Build history of the part. All positions in model axes, mm. Give positions to 0.01 mm unless a question says otherwise; leave off trailing zeros. Write each loop counter-clockwise with the first axis right and the second up, starting at its lowest first coordinate (ties: lowest second). Pieces come first, ordered by that corner, then holes.
from build123d import *

# Parameters (mm, degrees)
BOSS_EXTRUDE1_DEPTH = 1
BOSS_EXTRUDE2_DEPTH = 1.5
SKETCH3_W           = 70
SKETCH3_H           = 40
CUT_EXTRUDE1_DEPTH  = 10
SKETCH4_R           = 2.25
SKETCH4_R_2         = 3.25
CUT_EXTRUDE3_DEPTH  = 10


with BuildPart() as part:
    # Sketch1 → Boss-Extrude1 (new body)
    with BuildSketch(Plane.XY):
        Polygon((-85, 42), (85, 42), (86.5, 0), (85, -42), (-85, -42), (-86.5, 0), align=None)
    extrude(amount=BOSS_EXTRUDE1_DEPTH)

    # Sketch2 → Boss-Extrude2 (add)
    with BuildSketch(Plane.XY.offset(1)):
        Polygon((-83, 40.25), (83, 40.25), (84.5, 0), (83, -40.25), (-83, -40.25), (-84.5, 0), align=None)
    extrude(amount=BOSS_EXTRUDE2_DEPTH)

    # Sketch3 → Cut-Extrude1 (cut)
    with BuildSketch(Plane(origin=(0, 0, 0), x_dir=(-1, 0, 0), z_dir=(0, 0, -1))):
        with Locations((-27.5, 12)):
            Rectangle(SKETCH3_W, SKETCH3_H)
    extrude(amount=-CUT_EXTRUDE1_DEPTH, mode=Mode.SUBTRACT)

    # Sketch4 → Cut-Extrude3 (cut)
    with BuildSketch(Plane(origin=(0, 0, 0), x_dir=(-1, 0, 0), z_dir=(0, 0, -1))):
        with Locations((-65.954695658, -30.705934388)):
            Circle(SKETCH4_R)
        with Locations((-45.954695658, -30.705934388)):
            Circle(SKETCH4_R)
        with Locations((-9.054695658, -30.705934388)):
            Circle(SKETCH4_R)
        with Locations((10.945304342, -30.705934388)):
            Circle(SKETCH4_R)
        with Locations((47.845022936, -30.705934388)):
            Circle(SKETCH4_R)
        with Locations((67.845022936, -30.705934388)):
            Circle(SKETCH4_R)
        with Locations((67.845022936, -3.141963924)):
            Circle(SKETCH4_R)
        with Locations((47.845022936, -3.141963924)):
            Circle(SKETCH4_R)
        with Locations((57.845022936, 25.044065612)):
            Circle(SKETCH4_R_2)
    extrude(amount=-CUT_EXTRUDE3_DEPTH, mode=Mode.SUBTRACT)


solid = part.part
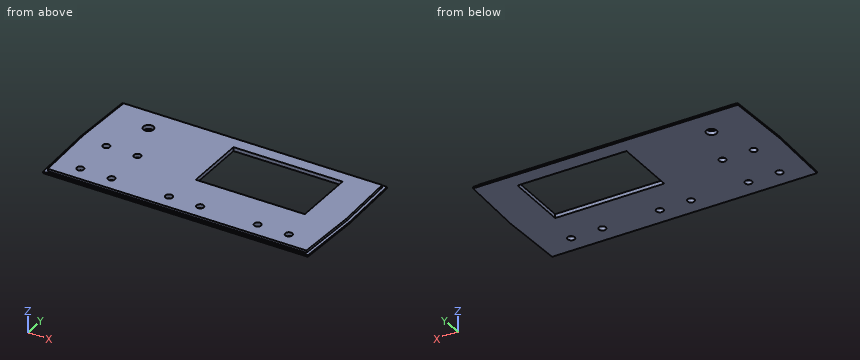
1. Drop flat-ended pins along their axis: pin 1 (0.8 mm diameter, centred on x = -26, z = 2, fed in from -Y); pin 2 (1 mm diameter, centred on x = 11.5, z = 2, fed in from +Y); pin 3 (0.8 mm diameter, centred on y = 6.5, z = 1.5, fed in from -X). Give the stop position or say it passes through.
2. Drill centre lines: line 1 along Y through (x, z) = (60.5, 1.65); line 2 along Y through (x, z) = (26.5, 0.6); line 3 along Y through (x, z) = (-68, 0.7). Where is each one in solid material? Low to high.
3. Saw through at C-C on y = -35. Give the cut face in (x, z), plus the area to 3 significant figures.
4. Saw through at D-D on y = 5.5. Give the cut face in (x, z), plus the area to 3 significant figures.
5. Saw through at A-A on z = 0.6. Count the separate pieces of the cut face and the enclosed holes in it, plus the area to 3 significant figures.
6. Saw through at B-B on y = 19. Give the cut face in (x, z), plus the area to 3 significant figures.
Outcome:
1. pin 1: stops at y = -40.25
1. pin 2: stops at y = 40.25
1. pin 3: stops at x = -84.27
2. line 1: y = -40.25 to -8, 32 to 40.25
2. line 2: y = -42 to -8, 32 to 42
2. line 3: y = -42 to -32.95, -28.46 to -5.39, -0.9 to 42
3. outline: (-85.25, 0) - (85.25, 0) - (85.25, 1) - (83.2, 1) - (83.2, 2.5) - (-83.2, 2.5) - (-83.2, 1) - (-85.25, 1) - close
3. area: 420 mm2
4. outline: (-86.3, 0) - (-7.5, 0) - (-7.5, 2.5) - (-84.3, 2.5) - (-84.3, 1) - (-86.3, 1) - close; (62.5, 0) - (86.3, 0) - (86.3, 1) - (84.3, 1) - (84.3, 2.5) - (62.5, 2.5) - close
4. area: 250 mm2
5. separate pieces: 1
5. enclosed holes: 10
5. area: 11,400 mm2
6. outline: (-85.82, 0) - (-7.5, 0) - (-7.5, 2.5) - (-83.79, 2.5) - (-83.79, 1) - (-85.82, 1) - close; (62.5, 0) - (85.82, 0) - (85.82, 1) - (83.79, 1) - (83.79, 2.5) - (62.5, 2.5) - close
6. area: 248 mm2
